Autodesk Inventor part; units mm, degrees
ref_plane "YZ Plane" through (0, 0, 0) normal (1, 0, 0) x (0, 1, 0)
ref_plane "XZ Plane" through (0, 0, 0) normal (0, 1, 0) x (-1, 0, 0)
ref_plane "XY Plane" through (0, 0, 0) normal (0, 0, 1) x (1, 0, 0)
sketch "Sketch1" plane through (0, 0, 0) normal (0, 1, 0) x (-1, 0, 0)
  line L0 (-132.08, -110.49) -> (132.08, -110.49)
  line L1 (132.08, -110.49) -> (132.08, 110.49)
  line L2 (132.08, 110.49) -> (-132.08, 110.49)
  line L3 (-132.08, 110.49) -> (-132.08, -110.49)
  line L4 (-132.08, -110.49) -> (132.08, 110.49) construction
  line L5 (132.08, -110.49) -> (-132.08, 110.49) construction
  point P0 (0, 0)
  dimension "d0" = 264.16
  dimension "d1" = 220.98
extrude "Extrusion1" add sketch "Sketch1" along normal blind 78.74
sketch "Sketch2" plane through (-132.08, 0, 110.49) normal (0, 0, 1) x (1, 0, 0)
  line L0 (264.16, 0) -> (264.16, 78.74)
  line L1 (0, 78.74) -> (264.16, 78.74)
  circle A0 centre (204.16, 39.37) radius 32.5
  point P0 (0, 0)
  point P1 (132.08, 0)
  dimension "d4" = 60
  dimension "d5" = 65
  dimension "d6" = 78.74
  dimension "d7" = 39.37
extrude "Extrusion2" add sketch "Sketch2" along normal blind 5
sketch "Sketch3" plane through (72.08, 39.37, 115.49) normal (0, 0, 1) x (1, 0, 0)
  circle A0 centre (0, 0) radius 32.5
  circle A1 centre (0, 0) radius 27.5
  point P0 (-72.08, -39.37)
  dimension "d10" = 55
extrude "Extrusion3" cut sketch "Sketch3" against normal blind 20 contours A1
fillet "Fillet1" radius 6 4 edges at (0, 78.74, 110.49) (0, 78.74, -110.49) (0, 0, -110.49) (0, 0, 110.49)
fillet "Fillet2" radius 1 16 edges at (-132.08, 76.9826, 108.7326) (-132.08, 78.74, 0) (-132.08, 76.9826, -108.7326) (-132.08, 39.37, -110.49) (-132.08, 1.7574, -108.7326) (-132.08, 0, 0) (-132.08, 1.7574, 108.7326) (-132.08, 39.37, 110.49) (132.08, 76.9826, -108.7326) (132.08, 39.37, -110.49) (132.08, 1.7574, -108.7326) (132.08, 0, 0) (132.08, 1.7574, 108.7326) (132.08, 39.37, 110.49) (132.08, 76.9826, 108.7326) (132.08, 78.74, 0)
equation "\"d7\" = 0.5 * d6"
properties part number "Projector-AcerP1500"
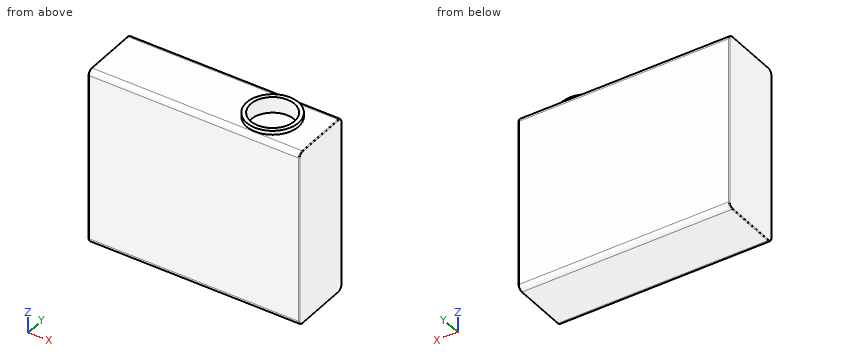
Part model, mm, in its own coordinate system. Coordinates: 2 decimals unless noted, no trailing zeros. Order: outer loops, then holes, each group sorted by start corner. A loop starts at its lowest first (then second) coordinate and runs counter-clockwise, first axis right, second up. Notation, with made-up numbers: M 30.25,11.25 L 44.25,11.25 A24 ccw 44.25,38.25 Z; hole C 51,57 d2. An arc over 180 degrees is marked long. Use a Markdown table: item, result.
(1) Cut at C-C on x = 72.08. Write the cut outline in (y, z).
A:
| item | result |
|---|---|
| outline | M 0,-104.49 A6 ccw 6,-110.49 L 72.74,-110.49 A6 ccw 78.74,-104.49 L 78.74,104.49 A6 ccw 72.74,110.49 L 71.87,110.49 L 71.87,115.49 L 66.87,115.49 L 66.87,95.49 L 11.87,95.49 L 11.87,115.49 L 6.87,115.49 L 6.87,110.49 L 6,110.49 A6 ccw 0,104.49 Z |
(2) Flat gauge pin, fed straight in: pin 1 (20 mm diameter, centred on x = -1, y = 42, fed in from +Z). Where does the tip first touch, or does it go through?
A:
| item | result |
|---|---|
| pin 1 | stops at z = 110.49 |
(3) Probe L1, parallel to X at y = 39, z = 109; L2, parallel to Y at x = 72.08, z = 110.75; L3, parallel to Y at x = 72, z = 102. List the from-to ranges inside material, lowest first.
A:
| item | result |
|---|---|
| L1 | x = -132.08 to 44.58, 99.58 to 132.08 |
| L2 | y = 6.87 to 11.87, 66.87 to 71.87 |
| L3 | y = 0 to 11.87, 66.87 to 78.74 |
(4) Cut at B-B on y = 39.37. Write the cut outline in (x, z), then the cut area to 3 significant figures.
A:
| item | result |
|---|---|
| outline | M -132.08,-109.49 A1 ccw -131.08,-110.49 L 131.08,-110.49 A1 ccw 132.08,-109.49 L 132.08,109.49 A1 ccw 131.08,110.49 L 104.58,110.49 L 104.58,115.49 L 99.58,115.49 L 99.58,95.49 L 44.58,95.49 L 44.58,115.49 L 39.58,115.49 L 39.58,110.49 L -131.08,110.49 A1 ccw -132.08,109.49 Z |
| area | 57,600 mm^2 |
(5) Cut at A-A on x = 28. Write the cut outline in (y, z).
A:
| item | result |
|---|---|
| outline | M 0,-104.49 A6 ccw 6,-110.49 L 72.74,-110.49 A6 ccw 78.74,-104.49 L 78.74,104.49 A6 ccw 72.74,110.49 L 6,110.49 A6 ccw 0,104.49 Z |
